Could you check a few things on this model? Use its own coordinates, in mm. Give positions to 0.01 mm unless a question says otherwise; leave off trailing zeros. Write each loop counter-clockwise with the first axis right and the second up, starting at its lowest first coordinate (ties: lowest second). Pieces come first, ordered by that corner, then holes. Notation, with made-up numbers: (-31.5, 60) - (0.5, 60) arc R30 ccw to (0.5, 90) - close; hole circle Ø9 at (79.25, 25). An arc over 180 degrees is marked (long way). Answer in a Markdown table with one row per item.
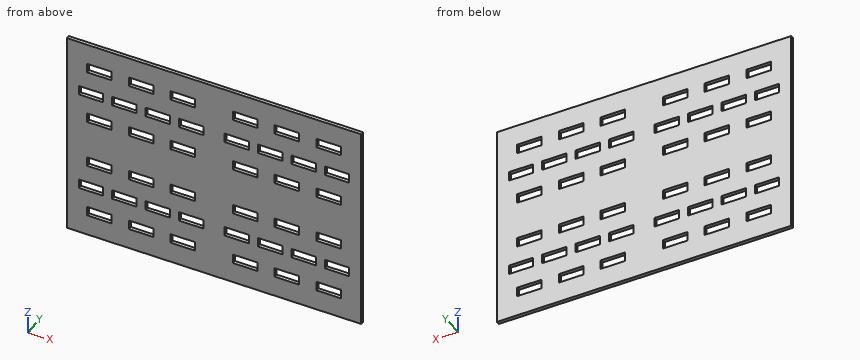
from build123d import *

# Parameters (mm, degrees)
F0_W     = 41
F0_H     = 15.5
F1_DEPTH = 3


with BuildPart() as f1:
    # F0 (on Front) → F1 (new body, symmetric)
    with BuildSketch(Plane.XZ):
        Polygon((-227.5, -172.5), (227.5, -172.5), (247.5, -172.5), (247.5, -152.5), (247.5, 152.5), (247.5, 172.5), (226.916667, 172.5), (-228.083333, 172.5), (-247.5, 172.5), (-247.5, 152.5), (-247.5, -152.5), (-247.5, -172.5), align=None)
        with Locations((-192.75, -130.125)):
            Rectangle(F0_W, F0_H, mode=Mode.SUBTRACT)
        with Locations((-122.5, -130.125)):
            Rectangle(F0_W, F0_H, mode=Mode.SUBTRACT)
        with Locations((-52.25, -130.125)):
            Rectangle(F0_W, F0_H, mode=Mode.SUBTRACT)
        with Locations((-206.8, -85)):
            Rectangle(F0_W, F0_H, mode=Mode.SUBTRACT)
        with Locations((-150.6, -85)):
            Rectangle(F0_W, F0_H, mode=Mode.SUBTRACT)
        with Locations((-192.75, -39.875)):
            Rectangle(F0_W, F0_H, mode=Mode.SUBTRACT)
        with Locations((-94.4, -85)):
            Rectangle(F0_W, F0_H, mode=Mode.SUBTRACT)
        with Locations((-38.2, -85)):
            Rectangle(F0_W, F0_H, mode=Mode.SUBTRACT)
        with Locations((-122.5, -39.875)):
            Rectangle(F0_W, F0_H, mode=Mode.SUBTRACT)
        with Locations((-52.25, -39.875)):
            Rectangle(F0_W, F0_H, mode=Mode.SUBTRACT)
        with Locations((52.25, -130.125)):
            Rectangle(F0_W, F0_H, mode=Mode.SUBTRACT)
        with Locations((122.5, -130.125)):
            Rectangle(F0_W, F0_H, mode=Mode.SUBTRACT)
        with Locations((192.75, -130.125)):
            Rectangle(F0_W, F0_H, mode=Mode.SUBTRACT)
        with Locations((38.2, -85)):
            Rectangle(F0_W, F0_H, mode=Mode.SUBTRACT)
        with Locations((94.4, -85)):
            Rectangle(F0_W, F0_H, mode=Mode.SUBTRACT)
        with Locations((52.25, -39.875)):
            Rectangle(F0_W, F0_H, mode=Mode.SUBTRACT)
        with Locations((122.5, -39.875)):
            Rectangle(F0_W, F0_H, mode=Mode.SUBTRACT)
        with Locations((150.6, -85)):
            Rectangle(F0_W, F0_H, mode=Mode.SUBTRACT)
        with Locations((206.8, -85)):
            Rectangle(F0_W, F0_H, mode=Mode.SUBTRACT)
        with Locations((192.75, -39.875)):
            Rectangle(F0_W, F0_H, mode=Mode.SUBTRACT)
        with Locations((-192.75, 39.875)):
            Rectangle(F0_W, F0_H, mode=Mode.SUBTRACT)
        with Locations((-206.8, 85)):
            Rectangle(F0_W, F0_H, mode=Mode.SUBTRACT)
        with Locations((-150.6, 85)):
            Rectangle(F0_W, F0_H, mode=Mode.SUBTRACT)
        with Locations((-122.5, 39.875)):
            Rectangle(F0_W, F0_H, mode=Mode.SUBTRACT)
        with Locations((-52.25, 39.875)):
            Rectangle(F0_W, F0_H, mode=Mode.SUBTRACT)
        with Locations((-94.4, 85)):
            Rectangle(F0_W, F0_H, mode=Mode.SUBTRACT)
        with Locations((-38.2, 85)):
            Rectangle(F0_W, F0_H, mode=Mode.SUBTRACT)
        with Locations((-192.75, 130.125)):
            Rectangle(F0_W, F0_H, mode=Mode.SUBTRACT)
        with Locations((-122.5, 130.125)):
            Rectangle(F0_W, F0_H, mode=Mode.SUBTRACT)
        with Locations((-52.25, 130.125)):
            Rectangle(F0_W, F0_H, mode=Mode.SUBTRACT)
        with Locations((52.25, 39.875)):
            Rectangle(F0_W, F0_H, mode=Mode.SUBTRACT)
        with Locations((122.5, 39.875)):
            Rectangle(F0_W, F0_H, mode=Mode.SUBTRACT)
        with Locations((38.2, 85)):
            Rectangle(F0_W, F0_H, mode=Mode.SUBTRACT)
        with Locations((94.4, 85)):
            Rectangle(F0_W, F0_H, mode=Mode.SUBTRACT)
        with Locations((192.75, 39.875)):
            Rectangle(F0_W, F0_H, mode=Mode.SUBTRACT)
        with Locations((150.6, 85)):
            Rectangle(F0_W, F0_H, mode=Mode.SUBTRACT)
        with Locations((206.8, 85)):
            Rectangle(F0_W, F0_H, mode=Mode.SUBTRACT)
        with Locations((52.25, 130.125)):
            Rectangle(F0_W, F0_H, mode=Mode.SUBTRACT)
        with Locations((122.5, 130.125)):
            Rectangle(F0_W, F0_H, mode=Mode.SUBTRACT)
        with Locations((192.75, 130.125)):
            Rectangle(F0_W, F0_H, mode=Mode.SUBTRACT)
    extrude(amount=F1_DEPTH, both=True)


solid = f1.part
1) Imagine slicing it at B-B (x = 159). List the corners of the cut face in (y, z) for me, then the cut area to 3 significant figures.
Check values:
| item | result |
|---|---|
| outline | (-3, -172.5) - (3, -172.5) - (3, -92.75) - (-3, -92.75) - close; (-3, -77.25) - (3, -77.25) - (3, 77.25) - (-3, 77.25) - close; (-3, 92.75) - (3, 92.75) - (3, 172.5) - (-3, 172.5) - close |
| area | 1,880 mm2 |
2) If I drill on line 1 (Z direction, x = -125, y = 2.5) (3 decimals); line 2 (Z direction, x = 85.5, y = -0.7), over which ranges is the centre line in solid material (lowest first)?
Check values:
| item | result |
|---|---|
| line 1 | z = -172.5 to -137.875, -122.375 to -47.625, -32.125 to 32.125, 47.625 to 122.375, 137.875 to 172.5 |
| line 2 | z = -172.5 to -92.75, -77.25 to 77.25, 92.75 to 172.5 |
3) Imagine slicing it at C-C (y = -1.7). State how many separate pieces and enclosed holes the cut face has, then the cut area to 3 significant figures.
Check values:
| item | result |
|---|---|
| separate pieces | 1 |
| enclosed holes | 40 |
| area | 145,000 mm2 |
4) Imagine slicing it at A-A (z = 128). List the corners of the cut face in (x, y) for me, then the cut area to 3 significant figures.
Check values:
| item | result |
|---|---|
| outline | (-247.5, -3) - (-213.25, -3) - (-213.25, 3) - (-247.5, 3) - close; (-172.25, -3) - (-143, -3) - (-143, 3) - (-172.25, 3) - close; (-102, -3) - (-72.75, -3) - (-72.75, 3) - (-102, 3) - close; (-31.75, -3) - (31.75, -3) - (31.75, 3) - (-31.75, 3) - close; (72.75, -3) - (102, -3) - (102, 3) - (72.75, 3) - close; (143, -3) - (172.25, -3) - (172.25, 3) - (143, 3) - close; (213.25, -3) - (247.5, -3) - (247.5, 3) - (213.25, 3) - close |
| area | 1,490 mm2 |
